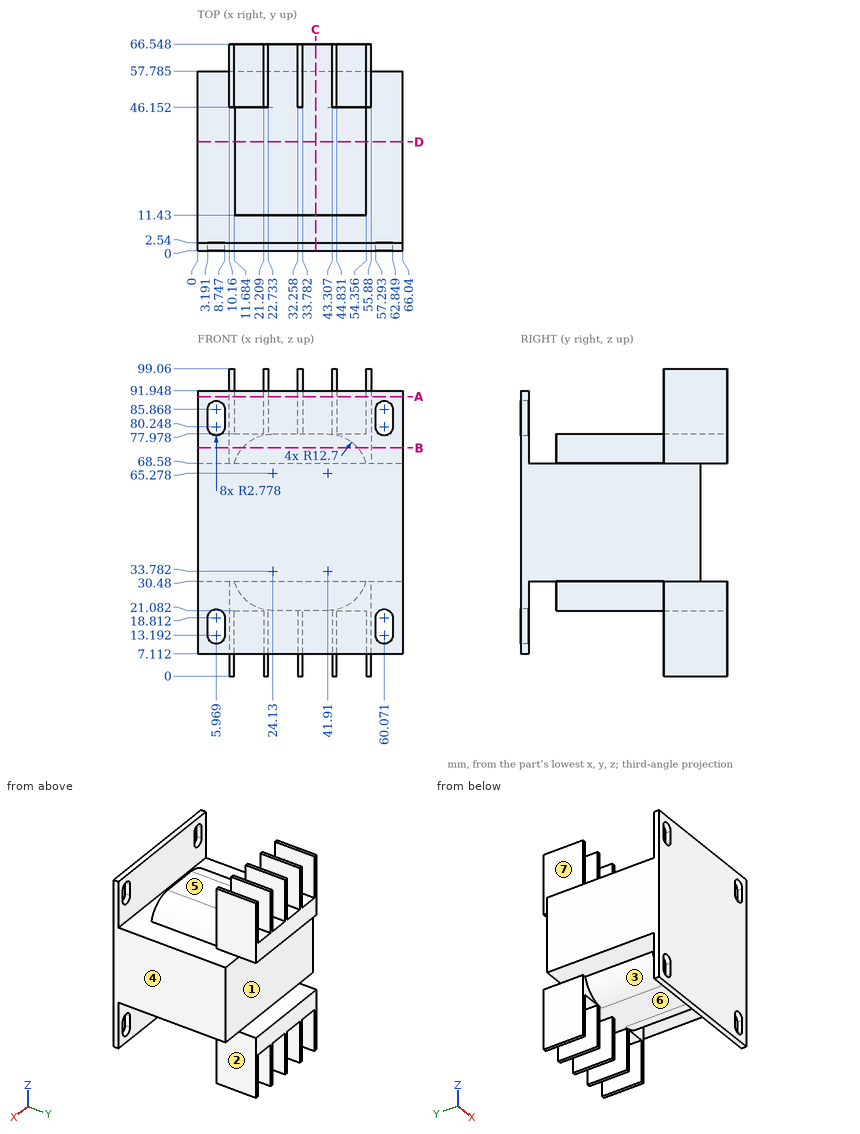
Input: dimensioned drawing with shaded views. Units: mm. Origin: part minimum x, y, z. A direction names the side the tool comes from. Coordinates: 2 decimals unless noted, no trailing zeros. Loops run counter-clockwise (first coordinate to the right, second up) from the corner with the lowest first, then second, coordinate; pieces in that order, holes last. Notation, with made-up numbers: M 17.5,-28.75 L 49.5,-28.75 A17 ccw 49.5,-23.75 Z; hole C 24.25,20.25 d9. An arc over 180 degrees is marked long. Use a Markdown table: item, result. Add a question column.
Q1. First-contact query: pin 1 (22.5 mm diameter, centred on y = 53, z = 88, fed in from +X); pin 2 (12 mm diameter, centred on y = 34.5, z = 34.5, fed in from -X); pin 3 (16.5 mm diameter, centred on y = 54, z = 10.5, fed in from -X); pin 4 (4 mm diameter, centred on x = 42, y = 42, fed in from -Z). Flat tips, straight axial feed; report the tip coordinate or a pass-through.
Q2. Section query A-A, the plane z = 90. Return loops of the section in (x, y).
Q3. Section query D-D, the plane y = 35. Return loops of the section in (x, z).
Q4. Material intervals for L1, parallel to Y at x = 20, z = 25.5; L2, parallel to Y at x = 25.5, z = 33.5 (3 decimals); L3, parallel to Z at x = 57.5, y = 24.5, sorted ascending.
Q5. Access query for the marked faces 1, 2 and 3. Directions: +Z, -Z, +X, -X, +Y, -Y. A direction counts if a zero-diameter tool reaches every point of the face in a straight line with its end or side. Return the directions, or none.
Q6. Draft query along X for the marked faces 4, 5, 6 and 7. Return one class per face: pulls with the +X half, pulls with the -X half, needs draft (parallel to the pull), parting line crosses it, or undercut.
Q7. Section query C-C, the plane x = 38. Return loops of the section in (y, z) (3 decimals), and give its area (3 significant figures).
Q8. Section query B-B, the plane z = 73.5. Return loops of the section in (x, y).
Result:
| question | item | result |
|---|---|---|
| 1 | pin 1 | stops at x = 55.88 |
| 1 | pin 2 | stops at x = 0 |
| 1 | pin 3 | stops at x = 10.16 |
| 1 | pin 4 | stops at z = 21.08 |
| 2 | outline | M 0,0 L 66.04,0 L 66.04,2.54 L 0,2.54 Z; M 10.16,46.15 L 11.68,46.15 L 11.68,66.55 L 10.16,66.55 Z; M 21.21,46.15 L 22.73,46.15 L 22.73,66.55 L 21.21,66.55 Z; M 32.26,46.15 L 33.78,46.15 L 33.78,66.55 L 32.26,66.55 Z; M 43.31,46.15 L 44.83,46.15 L 44.83,66.55 L 43.31,66.55 Z; M 54.36,46.15 L 55.88,46.15 L 55.88,66.55 L 54.36,66.55 Z |
| 3 | outline | M 0,30.48 L 11.87,30.48 A12.7 ccw 24.13,21.08 L 41.91,21.08 A12.7 ccw 54.17,30.48 L 66.04,30.48 L 66.04,68.58 L 54.17,68.58 A12.7 ccw 41.91,77.98 L 24.13,77.98 A12.7 ccw 11.87,68.58 L 0,68.58 Z |
| 4 | L1 | y = 0 to 2.54, 11.43 to 66.55 |
| 4 | L2 | y = 0 to 57.785 |
| 4 | L3 | z = 30.48 to 68.58 |
| 5 | face 1 | +X, -X, +Y |
| 5 | face 2 | -Z, +X, +Y |
| 5 | face 3 | -Z, -X |
| 6 | face 4 | pulls with the +X half |
| 6 | face 5 | undercut |
| 6 | face 6 | undercut |
| 6 | face 7 | pulls with the -X half |
| 7 | outline | M 0,7.112 L 2.54,7.112 L 2.54,30.48 L 11.43,30.48 L 11.43,21.082 L 66.548,21.082 L 66.548,30.48 L 57.785,30.48 L 57.785,68.58 L 66.548,68.58 L 66.548,77.978 L 11.43,77.978 L 11.43,68.58 L 2.54,68.58 L 2.54,91.948 L 0,91.948 Z |
| 7 | area | 3,360 mm2 |
| 8 | outline | M 0,0 L 66.04,0 L 66.04,2.54 L 0,2.54 Z; M 10.16,46.15 L 14.45,46.15 L 14.45,11.43 L 51.59,11.43 L 51.59,46.15 L 55.88,46.15 L 55.88,66.55 L 10.16,66.55 Z |
